```python
from build123d import *

# Parameters (mm, degrees)
SKETCH1_W           = 107.95
SKETCH1_H           = 12.7
BOSS_EXTRUDE1_DEPTH = 123.65
SKETCH2_R           = 3.175
CUT_EXTRUDE1_DEPTH  = 25.4
SKETCH4_R           = 1.985
CUT_EXTRUDE3_DEPTH  = 165.632363161
SKETCH6_R           = 2.6
CUT_EXTRUDE8_DEPTH  = 165.632363161


with BuildPart() as part:
    # Sketch1 → Boss-Extrude1 (new body)
    with BuildSketch(Plane.XY):
        with Locations((53.975, -6.35)):
            Rectangle(SKETCH1_W, SKETCH1_H)
    extrude(amount=BOSS_EXTRUDE1_DEPTH)

    # Sketch2 → Cut-Extrude1 (cut)
    with BuildSketch(Plane.XY.offset(123.65)):
        with Locations((19.05, -6.35)):
            Circle(SKETCH2_R)
        with Locations((88.9, -6.35)):
            Circle(SKETCH2_R)
    cut_extrude1 = extrude(amount=-CUT_EXTRUDE1_DEPTH, mode=Mode.SUBTRACT)

    # Mirror1: Cut-Extrude1 across plane
    add(cut_extrude1.mirror(Plane.XY.offset(61.825)), mode=Mode.SUBTRACT)

    # Sketch4 → Cut-Extrude3 (cut, through all)
    with BuildSketch(Plane(origin=(0, 0, 0), x_dir=(1, 0, 0), z_dir=(0, 1, 0))):
        with Locations(Location((9.135, -106.665, 0), (0, 0, 270))):
            Circle(SKETCH4_R)
        with Locations(Location((9.14, -16.99, 0), (0, 0, 270))):
            Circle(SKETCH4_R)
        with Locations(Location((98.81, -106.665, 0), (0, 0, 270))):
            Circle(SKETCH4_R)
        with Locations(Location((98.815, -16.99, 0), (0, 0, 270))):
            Circle(SKETCH4_R)
    extrude(amount=-CUT_EXTRUDE3_DEPTH, mode=Mode.SUBTRACT)

    # Sketch6 → Cut-Extrude8 (cut, through all)
    with BuildSketch(Plane(origin=(0, 0, 0), x_dir=(1, 0, 0), z_dir=(0, 1, 0))):
        with Locations(Location((32.275, -61.825, 0), (0, 0, 270))):
            Circle(SKETCH6_R)
        with Locations(Location((43.125, -43.032248738, 0), (0, 0, 270))):
            Circle(SKETCH6_R)
        with Locations(Location((64.825, -43.032248738, 0), (0, 0, 270))):
            Circle(SKETCH6_R)
        with Locations(Location((75.675, -61.825, 0), (0, 0, 270))):
            Circle(SKETCH6_R)
        with Locations(Location((64.825, -80.617751262, 0), (0, 0, 270))):
            Circle(SKETCH6_R)
        with Locations(Location((43.125, -80.617751262, 0), (0, 0, 270))):
            Circle(SKETCH6_R)
    extrude(amount=-CUT_EXTRUDE8_DEPTH, mode=Mode.SUBTRACT)


solid = part.part
```
CAD build for the part. Positions are in the model's coordinates, mm. A direction names the side the tool comes from. Coordinates: 2 decimals unless noted, no trailing zeros. Order: outer loops, then holes, each group sorted by start corner. A loop starts at its lowest first (then second) coordinate and runs counter-clockwise, first axis right, second up. Notation, with made-up numbers: (55, 31) - (104, 31) arc R33 ccw to (104, 63) - close; hole circle Ø11 at (-13, 1). An arc over 180 degrees is marked (long way). Answer in a Markdown table with one row per item.
1. Slice it at A-A, the plane z = 16.99. List the corners of the cut face in (x, y) (3 decimals), then the cut area to 3 significant figures.
Answer:
| item | result |
|---|---|
| outline | (0, -12.7) - (7.155, -12.7) - (7.155, 0) - (0, 0) - close; (11.125, -12.7) - (96.83, -12.7) - (96.83, 0) - (11.125, 0) - close; (100.8, -12.7) - (107.95, -12.7) - (107.95, 0) - (100.8, 0) - close; hole circle Ø6.35 at (19.05, -6.35); hole circle Ø6.35 at (88.9, -6.35) |
| area | 1,210 mm² |
2. Flat gauge pins, fed straight in: P1, Ø5, axis at x = 19.05, y = -6.35, coming from the +Z side; P2, Ø5.5, axis at x = 88.9, y = -6.35, coming from the -Z side. Where does each tip first touch, or does it go through?
Answer:
| item | result |
|---|---|
| P1 | z = 98.25 |
| P2 | z = 25.4 |
3. Pull direction Y, two halves, no side cores. Call faces 4 (the face through (53, 0, 61)), 5 (the face through (89, -6, 98.25)), 6 (the face through (53, -12.7, 61)), 7 (the face through (107.95, -6, 61)): +Y half, -Y half, draft (parallel to the pull), parting line (faces both ways), or undercut.
Answer:
| item | result |
|---|---|
| face 4 | +Y half |
| face 5 | undercut |
| face 6 | -Y half |
| face 7 | draft |
4. Slice it at B-B, the plane x = 88.9. List the corners of the cut face in (y, z) (3 decimals).
Answer:
| item | result |
|---|---|
| outline | (-12.7, 0) - (-9.525, 0) - (-9.525, 25.4) - (-3.175, 25.4) - (-3.175, 0) - (0, 0) - (0, 123.65) - (-3.175, 123.65) - (-3.175, 98.25) - (-9.525, 98.25) - (-9.525, 123.65) - (-12.7, 123.65) - close |
5. Drill centre lines: L1, parallel to Z at x = 65, y = -10.5; L2, parallel to Z at x = 63, y = -0.5; L3, parallel to Y at x = 19.05, z = 13 (3 decimals). Where is each one in solid material? Low to high. Write a range as from..to.
Answer:
| item | result |
|---|---|
| L1 | 0..40.44, 45.63..78.02, 83.21..123.65 |
| L2 | 0..41.18, 44.88..78.77, 82.47..123.65 |
| L3 | -12.7..-9.525, -3.175..0 |
6. 3-axis set-ups, long thin cutter, end or side, ignore diameter. For faces 1 (the face through (89, -6, 25.4)), 2 (the face through (15.88, -6.21, 111.13)), 3 (the face through (73.368, -6.261, 63.025)): which of +Z, -Z, +X, -X, +Y, -Y reach the whole face in a straight line?
Answer:
| item | result |
|---|---|
| face 1 | -Z |
| face 2 | +Z |
| face 3 | +Y, -Y |
7. Slice it at C-C, the plane y = -4.5. Give the number of separate pieces and of enclosed holes in the cut face, then the cut area to 3 significant figures.
Answer:
| item | result |
|---|---|
| separate pieces | 1 |
| enclosed holes | 10 |
| area | 12,600 mm² |
